```python
from build123d import *

# Parameters (mm, degrees)
F1_DEPTH = 160
F3_DEPTH = 5
F4_R     = 10.625
F5_DEPTH = 100
F6_R     = 3.75
F7_DEPTH = 50


with BuildPart() as f1:
    # F0 (on Top) → F1 (new body)
    with BuildSketch(Plane.XY):
        Polygon((6.928203, 12), (-6.928203, 12), (-13.856406, 0), (-6.928203, -12), (6.928203, -12), (13.856406, 0), align=None)
    extrude(amount=F1_DEPTH)

    # F2 (on Top) → F3 (join)
    with BuildSketch(Plane.XY):
        Polygon((-12.990381, -22.5), (12.990381, -22.5), (25.980762, 0), (12.990381, 22.5), (-12.990381, 22.5), (-25.980762, 0), align=None)
    extrude(amount=F3_DEPTH)

    # F4 (on face) → F5 (cut)
    with BuildSketch(Plane.XY.offset(160)):
        Polygon((6.928203, 12), (-6.928203, 12), (-13.856406, 0), (-6.928203, -12), (6.928203, -12), (13.856406, 0), align=None)
        Circle(F4_R, mode=Mode.SUBTRACT)
    extrude(amount=-F5_DEPTH, mode=Mode.SUBTRACT)

    # F6 (on Front) → F7 (cut, symmetric)
    with BuildSketch(Plane.XZ):
        with Locations((0, 70)):
            Circle(F6_R)
    extrude(amount=F7_DEPTH, both=True, mode=Mode.SUBTRACT)


solid = f1.part
```
Source: CAD feature listing. Evaluate the final solid. Frame: model axes, mm. A direction names the side the tool comes from. Give positions to 0.01 mm unless a question says otherwise; leave off trailing zeros. Loops run counter-clockwise (first coordinate to the right, second up) from the corner with the lowest first, then second, coordinate; pieces in that order, holes last. Notation, with made-up numbers: (9, 22) -> (56, 22) arc R22 cw to (56, 49) -> close; hole circle Ø4 at (-18, 12). An arc over 180 degrees is marked (long way). Use a Markdown table: item, result. Add a question column.
(1) Pull-direction query (Z, two-part tool) for faces 1 (the face through (-0.488, -0.149, 73.718)), 2 (the face through (11.2, 5.3, 5)), 3 (the face through (19.58, 11.09, 2.46)); classes: +Z half, -Z half, draft (parallel to the pull), parting line (faces both ways), or undercut.
(2) Section query A-A (x = 0). Output: boundary loops of the cut face in (y, z) (3 decimals).
(3) Section query B-B (z = 44). Output: boundary loops of the cut face in (x, y).
(4) Access query for faces 4 (the face through (0, 12, 32)), 5 (the face through (-8.43, -6.47, 110.7)), 6 (the face through (0, -12, 32)), 7 (the face through (10.344, -6.084, 32.115)). Directions: +Z, -Z, +X, -X, +Y, -Y. A direction counts if a zero-diameter tool reaches every point of the face in a straight line with its end or side. Return the directions, or none.
(5) Section query C-C (y = 3.5). Output: boundary loops of the cut face in (x, z).
(6) Ray query, line 1 (Z direction, x = 0, y = -5); line 2 (X direction, y = 2.25, z = 70); line 3 (X direction, y = 7, z = 68). Return the intervals inside material, ascending.
(7) Section query D-D (z = 70). Output: boundary loops of the cut face in (x, y) (3 decimals).
(8) First-contact query: pin 1 Ø12 at (y, z) = (9, 131.5) entering from -X; pin 2 Ø15 at (x, z) = (-1, 46) entering from -Y; pin 3 Ø6 at (x, z) = (19.5, 52.5) entering from +Y; pin 4 Ø4 at (x, z) = (-3.5, 37) entering from +Y. Flat tips, straight axial feed; report the tip coordinate or a pass-through.
Checked values:
| question | item | result |
|---|---|---|
| 1 | face 1 | undercut |
| 1 | face 2 | +Z half |
| 1 | face 3 | draft |
| 2 | outline | (-22.5, 0) -> (22.5, 0) -> (22.5, 5) -> (12, 5) -> (12, 60) -> (10.625, 60) -> (10.625, 66.25) -> (-10.625, 66.25) -> (-10.625, 60) -> (-12, 60) -> (-12, 5) -> (-22.5, 5) -> close; (-10.625, 73.75) -> (10.625, 73.75) -> (10.625, 160) -> (-10.625, 160) -> close |
| 3 | outline | (-13.86, 0) -> (-6.93, -12) -> (6.93, -12) -> (13.86, 0) -> (6.93, 12) -> (-6.93, 12) -> close |
| 4 | face 4 | +Z, +X, -X, +Y |
| 4 | face 5 | +Z |
| 4 | face 6 | +Z, +X, -X, -Y |
| 4 | face 7 | +Z, +X, -Y |
| 5 | outline | (-23.96, 0) -> (23.96, 0) -> (23.96, 5) -> (11.84, 5) -> (11.84, 60) -> (10.03, 60) -> (10.03, 160) -> (-10.03, 160) -> (-10.03, 60) -> (-11.84, 60) -> (-11.84, 5) -> (-23.96, 5) -> close; hole circle Ø7.5 at (0, 70) |
| 6 | line 1 | 0 to 66.25, 73.75 to 160 |
| 6 | line 2 | -10.38 to -3.75, 3.75 to 10.38 |
| 6 | line 3 | -7.99 to -3.17, 3.17 to 7.99 |
| 7 | outline | (-3.75, -9.941) -> (-3.75, 9.941) arc R10.625 ccw to start; (3.75, -9.941) arc R10.625 ccw to (3.75, 9.941) -> close |
| 8 | pin 1 | x = -10.19 |
| 8 | pin 2 | y = -12 |
| 8 | pin 3 | through |
| 8 | pin 4 | y = 12 |
